For this review, use the dimensioned drawing (mm, ordinates from the lowest corner) and the shaded views. Give positions to 0.01 mm unless a question says otherwise; leave off trailing zeros. Order: outer loops, then holes, each group sorted by start corner. A loop starts at its lowest first (then second) coordinate and runs counter-clockwise, first axis right, second up.
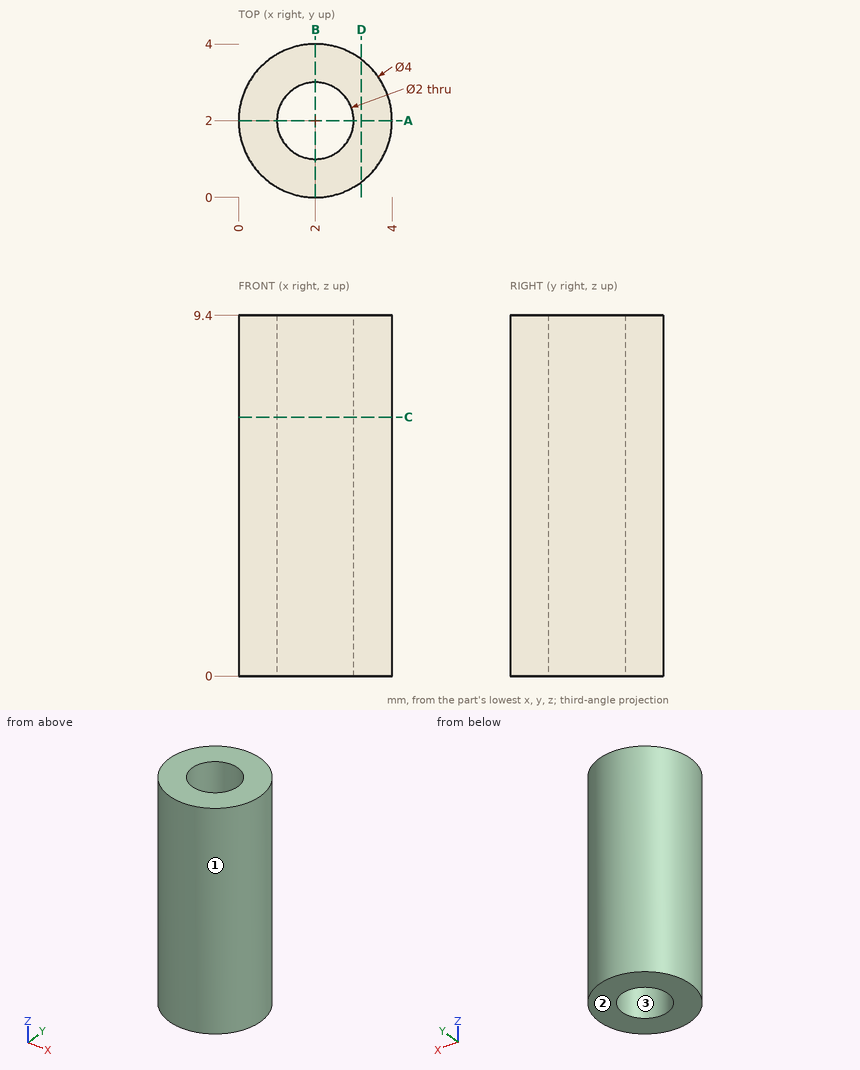
1. Insertion check: pin 1 (1.5 mm diameter, centred on x = 0.5, y = 2, fed in from -Z); pin 2 (2 mm diameter, centred on y = 3.5, z = 6, fed in from +X); pin 3 (1.8 mm diameter, centred on x = 2, y = 2, fed in from +Z); pin 4 (1 mm diameter, centred on x = 0.5, z = 4.5, fed in from -Y). Each pin has a flat end and moves straight along its axis. Give the tip position at first contact, or say it passes through.
2. To check wall thickness, follow line 1 (Y direction, x = 2, z = 5.25); line 2 (X direction, y = 1.7, z = 1); line 3 (X direction, y = 2.9, z = 5). State the ranges of each line that lie inside material, in increasing order.
3. Draft analysis for pull direction X (two halves, no side actions). For the marked faces 1, 2 and 3, state which applies: pulls with the +X half, pulls with the -X half, needs draft (parallel to the pull), parting line crosses it, or undercut.
4. Take a section at D-D (x = 3.2). Write out the cut boundary in (y, z).
5. Take a section at C-C (z = 6.75). Write out the cut boundary in (x, y).
6. Take a section at A-A (y = 2). Write out the cut boundary in (x, z).
Answer:
1. pin 1: stops at z = 0
1. pin 2: stops at x = 3.94
1. pin 3: passes through
1. pin 4: stops at y = 0.27
2. line 1: y = 0 to 1, 3 to 4
2. line 2: x = 0.02 to 1.05, 2.95 to 3.98
2. line 3: x = 0.21 to 1.56, 2.44 to 3.79
3. face 1: parting line crosses it
3. face 2: needs draft
3. face 3: undercut
4. outline: (0.4, 0) - (3.6, 0) - (3.6, 9.4) - (0.4, 9.4) - close
5. outline: circle Ø4 at (2, 2); hole circle Ø2 at (2, 2)
6. outline: (0, 0) - (1, 0) - (1, 9.4) - (0, 9.4) - close; (3, 0) - (4, 0) - (4, 9.4) - (3, 9.4) - close
